Work out the finished part from the listing and answer in its coordinate system (mm). A direction names the side the tool comes from. Coordinates: 2 decimals unless noted, no trailing zeros. Order: outer loops, then holes, each group sorted by start corner. A loop starts at its lowest first (then second) coordinate and runs counter-clockwise, first axis right, second up. Notation, with made-up numbers: (24, -25.5) -> (51, -25.5) arc R12 ccw to (51, -12.5) -> close; hole circle Ø1 at (84, 36). An arc over 180 degrees is marked (long way). Write item = value, one per line. Start each with the question number.
Q1. The part is cut by section B-B, the plane y = 6. Determine the outline of the cut face in (x, z), plus the area to 3 significant figures.
Q2. For a pull along Z with two mould halves and no side action, classify faces 3 (the flat face through (-21, 0, 8)), 4 (the cylindrical face through (-30.79, -3.32, 0.74)), 5 (the flat face through (4, 0.11, 0.11)) as +Z half, -Z half, draft (parallel to the pull), parting line (faces both ways), or undercut.
Q3. The part is cut by section A-A, the plane x = -35. Determine the outline of the cut face in (y, z), plus the area to 3 significant figures.
Q4. Which of the six approach directions +Z, -Z, +X, -X, +Y, -Y give full straight-line access (tool end or side, diameter ignored) to faces 1 (the flat face through (7.18, -0.06, 15.28)), 2 (the conical face through (-14.312, -0.576, -0.128))?
Q5. Flat-ended cylindrical pins translate along their axes: pin 1 (1 mm diameter, centred on x = -13, y = -1.5, fed in from -Z); pin 2 (2 mm diameter, centred on x = -0.5, y = 4, fed in from +Z); pin 3 (5 mm diameter, centred on x = 13.5, y = -3, fed in from +Z). Find the tip coordinate at first contact, or state that the pin passes through.
Q6. Straight lines are drawn through the part: L1, parallel to Z at x = -23, y = 0; L2, parallel to Z at x = 0.5, y = 4.75. For each, find the intervals that lie inside material, in ascending order. Write a range as from..to.
```python
from build123d import *

# Parameters (mm, degrees)
SKETCH2_R             = 4
SKETCH3_W             = 50
SKETCH3_H             = 16
BOSS_EXTRUDE1_DEPTH   = 8
M8_TAPPED_HOLE1_D     = 6.8
M8_TAPPED_HOLE1_DEPTH = 30
M8_TAPPED_HOLE1_TIP   = 2.042926105


with BuildPart() as part:
    # Sweep1: sweep along a path in Sketch1
    with BuildLine(Plane(origin=(0, 0, 0), x_dir=(1, 0, 0), z_dir=(0, 1, 0))) as sweep1_path:
        ThreePointArc((7.144247806, -15.320888862), (38.126155741, 8.452365235), (0, 0))
    # Sketch2 → Sweep1 (sweep)
    with BuildSketch(Plane.XY):
        Circle(SKETCH2_R)
    sweep(path=sweep1_path.line)

    # Sketch3 → Boss-Extrude1 (add, symmetric)
    with BuildSketch(Plane(origin=(0, 0, 0), x_dir=(1, 0, 0), z_dir=(0, 1, 0))):
        with Locations((-21, 0)):
            Rectangle(SKETCH3_W, SKETCH3_H)
    extrude(amount=BOSS_EXTRUDE1_DEPTH, both=True)

    # M8 Tapped Hole1
    with Locations(Plane.ZY.offset(46)):
        with Locations((0, 0)):
            Hole(M8_TAPPED_HOLE1_D / 2, depth=M8_TAPPED_HOLE1_DEPTH)
            with Locations((0, 0, -(M8_TAPPED_HOLE1_DEPTH + M8_TAPPED_HOLE1_TIP / 2))):  # 118° drill point
                Cone(0, M8_TAPPED_HOLE1_D / 2, M8_TAPPED_HOLE1_TIP, mode=Mode.SUBTRACT)


solid = part.part
```
Model answer:
q1.outline = (-46, -8) -> (4, -8) -> (4, 8) -> (-46, 8) -> close
q1.area = 800 mm2
q2.face_3 = +Z half
q2.face_4 = undercut
q2.face_5 = draft
q3.outline = (-8, -8) -> (8, -8) -> (8, 8) -> (-8, 8) -> close; hole circle Ø6.8 at (0, 0)
q3.area = 220 mm2
q4.face_1 = -X, +Y, -Y
q4.face_2 = -X
q5.pin_1 = -8
q5.pin_2 = 8
q5.pin_3 = 23.34
q6.L1 = -8..-3.4, 3.4..8
q6.L2 = -8..8
